from build123d import *

# Parameters (mm, degrees)
F0_R     = 50
F1_DEPTH = 100
F2_R     = 60
F3_DEPTH = 5
F4_R     = 1


with BuildPart() as f1:
    # F0 (on Top) → F1 (new body)
    with BuildSketch(Plane.XY):
        Circle(F0_R)
    extrude(amount=F1_DEPTH)

    # F2 (on face) → F3 (join)
    with BuildSketch(Plane.XY.offset(100)):
        Circle(F2_R)
    extrude(amount=-F3_DEPTH)

    # F4
    f4_edges = [f1.edges().sort_by_distance(p)[0] for p in [
        (60, 0, 97.5),
        (-60, 0, 100),
        (-60, 0, 95),
    ]]
    fillet(f4_edges, radius=F4_R)


solid = f1.part
The model under review builds one solid part; all positions refer to its coordinate system, in mm. A direction names the side the tool comes from. Round coordinates to 2 decimals unless told otherwise and drop trailing zeros. Order: outer loops, then holes, each group sorted by start corner. A loop starts at its lowest first (then second) coordinate and runs counter-clockwise, first axis right, second up. Notation, with made-up numbers: (53, 73) - (71, 73) arc R16 ccw to (71, 89) - close; hole circle Ø3 at (-36.5, -31). An arc over 180 degrees is marked (long way). Use one line per item in the form item = value.
Q1. Clearance check with flat-ended pins moving along their axes: P1, Ø10, axis at y = 4.5, z = 83, coming from the -X side; P2, Ø10, axis at y = 32, z = 36, coming from the -X side; P3, Ø5, axis at x = -35.5, z = 41.5, coming from the -Y side. State where each tip first meets the part, or that it passes through.
Response values:
P1 = -50
P2 = -42.08
P3 = -37.56
Q2. To check wall thickness, follow line 1 (Z direction, x = 45, y = -22); line 2 (X direction, y = -26.5, z = 25.5); line 3 (X direction, y = -23.5, z = 66.5). State the ranges of each line that lie inside material, in increasing order.
Response values:
line_1 = 95 to 100
line_2 = -42.4 to 42.4
line_3 = -44.13 to 44.13
Q3. Tool access review of faces 1 (the flat face through (-48.35, 13.39, 95)), 2 (the cylindrical face through (-59.94, 2.64, 97.52)): name each direction out of +Z, -Z, +X, -X, +Y, -Y from which nothing blocks a thin tool from reaching the whole face with its end or side.
Response values:
face_1 = -Z
face_2 = +Z, -Z
Q4. Add section A-A on y = 0. Give the boundary of the cut face in (x, z).
Response values:
outline = (-60, 96) arc R1 ccw to (-59, 95) - (-50, 95) - (-50, 0) - (50, 0) - (50, 95) - (59, 95) arc R1 ccw to (60, 96) - (60, 99) arc R1 ccw to (59, 100) - (-59, 100) arc R1 ccw to (-60, 99) - close
Q5. Add section C-C on z = 70.5. Give the boundary of the cut face in (x, y).
Response values:
outline = circle Ø100 at (0, 0)
